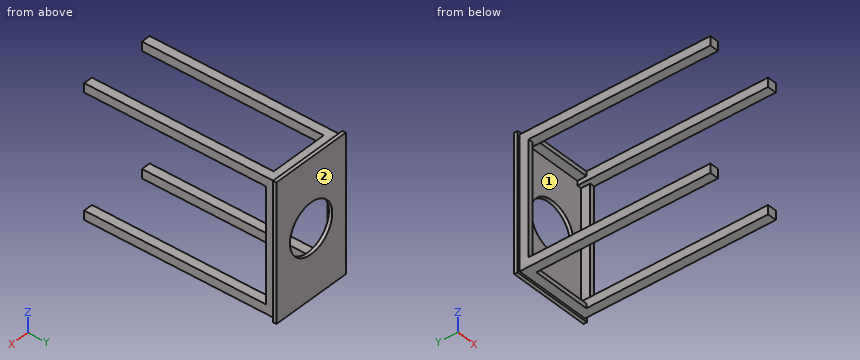
Autodesk Inventor part; units mm, degrees
ref_plane "YZ Plane" through (0, 0, 0) normal (1, 0, 0) x (0, 1, 0)
ref_plane "XZ Plane" through (0, 0, 0) normal (0, 1, 0) x (-1, 0, 0)
ref_plane "XY Plane" through (0, 0, 0) normal (0, 0, 1) x (1, 0, 0)
sketch "Sketch1" plane through (0, 0, 0) normal (0, 1, 0) x (-1, 0, 0)
  line L0 (457.2, 762) -> (-457.2, 762)
  line L1 (-457.2, 762) -> (-457.2, -762)
  line L2 (-457.2, -762) -> (457.2, -762)
  line L3 (457.2, -762) -> (457.2, 762)
  line L4 (457.2, 762) -> (-457.2, -762) construction
  line L5 (-457.2, 762) -> (457.2, -762) construction
  point P0 (0, 0)
  dimension "d0" = 914.4
  dimension "d1" = 1524
extrude "Extrusion1" add sketch "Sketch1" along normal blind 38.1
sketch "Sketch2" plane through (0, 0, 0) normal (0, -1, 0) x (1, 0, 0)
  line L0 (-381, 685.8) -> (381, 685.8) construction
  line L1 (381, 685.8) -> (381, -685.8) construction
  line L2 (381, -685.8) -> (-381, -685.8) construction
  line L3 (-381, -685.8) -> (-381, 685.8) construction
  line L4 (-381, 685.8) -> (381, -685.8) construction
  line L5 (381, 685.8) -> (-381, -685.8) construction
  line L6 (330.2, 736.6) -> (431.8, 736.6)
  line L7 (431.8, 736.6) -> (431.8, 635)
  line L8 (431.8, 635) -> (330.2, 635)
  line L9 (330.2, 635) -> (330.2, 736.6)
  line L10 (330.2, 736.6) -> (431.8, 635) construction
  line L11 (431.8, 736.6) -> (330.2, 635) construction
  line L12 (431.8, -635) -> (330.2, -635)
  line L13 (330.2, -635) -> (330.2, -736.6)
  line L14 (330.2, -736.6) -> (431.8, -736.6)
  line L15 (431.8, -736.6) -> (431.8, -635)
  line L16 (431.8, -635) -> (330.2, -736.6) construction
  line L17 (330.2, -635) -> (431.8, -736.6) construction
  line L18 (-431.8, -736.6) -> (-330.2, -736.6)
  line L19 (-330.2, -736.6) -> (-330.2, -635)
  line L20 (-330.2, -635) -> (-431.8, -635)
  line L21 (-431.8, -635) -> (-431.8, -736.6)
  line L22 (-431.8, -736.6) -> (-330.2, -635) construction
  line L23 (-330.2, -736.6) -> (-431.8, -635) construction
  line L24 (-431.8, 736.6) -> (-330.2, 736.6)
  line L25 (-330.2, 736.6) -> (-330.2, 635)
  line L26 (-330.2, 635) -> (-431.8, 635)
  line L27 (-431.8, 635) -> (-431.8, 736.6)
  line L28 (-431.8, 736.6) -> (-330.2, 635) construction
  line L29 (-330.2, 736.6) -> (-431.8, 635) construction
  point P0 (0, 0)
  dimension "d6" = 762
  dimension "d7" = 1371.6
  dimension "d8" = 101.6
  dimension "d9" = 101.6
  dimension "d10" = 101.6
  dimension "d11" = 101.6
  dimension "d12" = 101.6
  dimension "d13" = 101.6
  dimension "d14" = 101.6
  dimension "d15" = 101.6
extrude "Extrusion2" add sketch "Sketch2" along normal blind 2133.6
sketch "Sketch3" plane through (0, 0, 0) normal (0, -1, 0) x (1, 0, 0)
  line L0 (431.8, 635) -> (330.2, 635)
  line L1 (431.8, 635) -> (381, 635)
  line L2 (381, 635) -> (381, -635)
  line L3 (381, -635) -> (431.8, -635)
  line L4 (431.8, -635) -> (431.8, 635)
  line L5 (0, 0) -> (0, -69.3079) construction
  line L6 (-431.8, 635) -> (-330.2, 635)
  line L7 (-431.8, 635) -> (-381, 635)
  line L8 (-381, 635) -> (-381, -635)
  line L9 (-381, -635) -> (-431.8, -635)
  line L10 (-431.8, -635) -> (-431.8, 635)
  line L11 (330.2, -736.6) -> (330.2, -635)
  line L12 (-330.2, -736.6) -> (330.2, -736.6)
  line L13 (330.2, -736.6) -> (330.2, -685.8)
  line L14 (330.2, -685.8) -> (-330.2, -685.8)
  line L15 (-330.2, -685.8) -> (-330.2, -736.6)
  line L16 (0, 0) -> (54.1332, 0) construction
  line L17 (330.2, 736.6) -> (330.2, 635)
  line L18 (-330.2, 736.6) -> (330.2, 736.6)
  line L19 (330.2, 736.6) -> (330.2, 685.8)
  line L20 (330.2, 685.8) -> (-330.2, 685.8)
  line L21 (-330.2, 685.8) -> (-330.2, 736.6)
  dimension "d18" = 50.8
  dimension "d19" = 1270
  dimension "d20" = 50.8
extrude "Extrusion3" add sketch "Sketch3" along normal blind 101.6
sketch "Sketch4" plane through (0, 38.1, 0) normal (0, 1, 0) x (1, 0, 0)
  circle A0 centre (0, 0) radius 279.4
  dimension "d23" = 558.8
extrude "Extrusion4" cut sketch "Sketch4" against normal blind 101.6
properties part number "table" material "Laminated Veneer Lumber"
Can you work these out from the model? Positions are in its coordinate system, mm. Face numbers are marked on the shaded views. Coordinates: 2 decimals unless noted, no trailing zeros. Loops run counter-clockwise (first coordinate to the right, second up) from the corner with the lowest first, then second, coordinate; pieces in that order, holes last. Notation, with made-up numbers: M 43,53.5 L 66,53.5 A11 cw 66,74.5 Z; hole C -38.75,14.5 d8. An arc over 180 degrees is marked long. Answer as CSV lines item,"result". Start each with the question number.
1. Suppose I cut it at B-B, the plane y = -1789.5. List the corners of the cut face in (x, z) for me.
2. Suppose I cut it at C-C, the plane x = 0. List the corners of the cut face in (y, z) for me.
3. Suppose I cut it at D-D, the plane x = 356. List the corners of the cut face in (y, z) for me.
4. Thinking about a two-plate mould opening in Z: for the marked faces 1 and 2, which applies, +Z half, -Z half, draft (parallel to the pull), parting line (faces both ways), or undercut?
5. For pin 1 Ø15 at (x, z) = (403.5, 295) entering from -Y, with a flat end and sliding along its axis, tell me the tip position at first contact or that it passes through.
6. If I drill on probe 1 along X at (y, z) = (-88, 18); probe 2 along Z at (x, y) = (408, -317.5); probe 3 along X at (y, z) = (28, 0), over which ranges is the centre line in solid material (lowest first)? Write a range as [from, to].
7. Suppose I cut it at A-A, the plane z = 0. List the corners of the cut face in (x, y) for me.
Output:
1,outline,"M -431.8,-736.6 L -330.2,-736.6 L -330.2,-635 L -431.8,-635 Z; M -431.8,635 L -330.2,635 L -330.2,736.6 L -431.8,736.6 Z; M 330.2,-736.6 L 431.8,-736.6 L 431.8,-635 L 330.2,-635 Z; M 330.2,635 L 431.8,635 L 431.8,736.6 L 330.2,736.6 Z"
2,outline,"M -101.6,-736.6 L 0,-736.6 L 0,-762 L 38.1,-762 L 38.1,-279.4 L 0,-279.4 L 0,-685.8 L -101.6,-685.8 Z; M -101.6,685.8 L 0,685.8 L 0,279.4 L 38.1,279.4 L 38.1,762 L 0,762 L 0,736.6 L -101.6,736.6 Z"
3,outline,"M -2133.6,-736.6 L 0,-736.6 L 0,-762 L 38.1,-762 L 38.1,762 L 0,762 L 0,736.6 L -2133.6,736.6 L -2133.6,635 L 0,635 L 0,-635 L -2133.6,-635 Z"
4,face 1,"undercut"
4,face 2,"draft"
5,pin 1,"stops at y = -101.6"
6,probe 1,"x = [-431.8, -381], [381, 431.8]"
6,probe 2,"z = [-736.6, -635], [635, 736.6]"
6,probe 3,"x = [-457.2, -279.4], [279.4, 457.2]"
7,outline,"M -457.2,0 L -431.8,0 L -431.8,-101.6 L -381,-101.6 L -381,0 L -279.4,0 L -279.4,38.1 L -457.2,38.1 Z; M 279.4,0 L 381,0 L 381,-101.6 L 431.8,-101.6 L 431.8,0 L 457.2,0 L 457.2,38.1 L 279.4,38.1 Z"
